For this review, take the finished solid that the model builds, in its own axes (mm). Face numbers are marked on the shaded views. A direction names the side the tool comes from. Round coordinates to 2 decimals unless told otherwise and drop trailing zeros. Loops run counter-clockwise (first coordinate to the right, second up) from the corner with the lowest first, then second, coordinate; pieces in that order, holes last. Notation, with made-up numbers: (-39, -3) -> (-26, -3) arc R26 cw to (-26, 14) -> close; hole circle Ø8 at (65, 25). An arc over 180 degrees is marked (long way). One line per question, with ' | ' between items. Start each with the question number.
1. For the marked faces 1, 2, 3 and 4, list the 3-axis set-ups (+Z, -Z, +X, -X, +Y, -Y) from which the entire face can be reached by the end or side of a thin tool; tool diameter is ignored.
2. Consider section B-B (z = 45). Write out the cut boundary in (x, y), and give its area (3 significant figures).
3. Consider section D-D (y = 25.5). Write out the cut boundary in (x, z), and give its area (3 significant figures).
4. Consider section A-A (y = 78). Write out the cut boundary in (x, z), and give its area (3 significant figures).
5. Wall thickness on line 1 along Z through (x, y) = (-76, 15.5); line 2 along X through (y, z) = (-24, 123); line 3 along Y through (x, z) = (-68, 65.5): over which ranges is each line inside the solid? List them lowest first.
6. For pin 1 Ø10 at (y, z) = (64.5, 103.5) entering from +X; pin 2 Ø4.5 at (x, y) = (-5.5, 86) entering from -Z; pin 3 Ø5 at (y, z) = (56.5, 121.5) entering from -X, all flat-tipped, find the tip position at first contact; note any pin that passes through.
7. Consider section C-C (z = 67.5). Write out the cut boundary in (x, y), and give its area (3 significant figures).
```python
from build123d import *

# Parameters (mm, degrees)
BOSS_EXTRUDE1_DEPTH = 150
BOSS_EXTRUDE2_REACH = 243.582
SKETCH2_W           = 54.603647952
SKETCH2_H           = 44.432380196
BOSS_EXTRUDE3_REACH = 243.582
SKETCH2_3_W         = 54.603647952
SKETCH2_3_H         = 44.432380196
MIRROR1_START       = 47.698176024
MIRROR1_DEPTH       = 54.603647952
CUT_EXTRUDE1_DEPTH  = 194.302477267
CUT_EXTRUDE2_DEPTH  = 54.603647952
BOSS_EXTRUDE4_START = -100
BOSS_EXTRUDE4_DEPTH = 10


# Read off the part's stored shape, not the designer's step: Mirror1
with BuildPart() as part:
    # Sketch1 → Boss-Extrude1 (new body)
    with BuildSketch(Plane.XY):
        Polygon((-42.309401077, 73.282032303), (-84.618802154, 0), (-63.464101615, -36.641016151), (-60, -34.641016151), (-80, 0), (-40, 69.282032303), (40, 69.282032303), (80, 0), (60, -34.641016151), (63.464101615, -36.641016151), (84.618802154, 0), (42.309401077, 73.282032303), align=None)
    extrude(amount=BOSS_EXTRUDE1_DEPTH)

    # Boss-Extrude2: up to this face of the body (flat: up to its plane)
    boss_extrude2_end = Plane(part.part.faces().sort_by_distance((74.041451884, -18.320508076, 75))[0])
    # Sketch2 → Boss-Extrude2 (add, up to the picked face)
    with BuildSketch(Plane(origin=(90, 0, 0), x_dir=(0, 0, -1), z_dir=(1, 0, 0)), mode=Mode.PRIVATE) as boss_extrude2_sk1:
        with Locations((-75, 0)):
            Rectangle(SKETCH2_W, SKETCH2_H)
    boss_extrude2_tool1 = split(extrude(boss_extrude2_sk1.sketch, amount=-BOSS_EXTRUDE2_REACH, mode=Mode.PRIVATE), bisect_by=boss_extrude2_end, keep=Keep.BOTH, mode=Mode.PRIVATE)
    add(boss_extrude2_tool1.solids().sort_by(Axis((90, 0, 75), (-1, 0, 0)))[0])

    # Boss-Extrude3: up to this face of the body (flat: up to its plane)
    boss_extrude3_end = Plane(part.part.faces().sort_by_distance((63.464101615, 36.641016151, 75))[0])
    # Sketch2<3> → Boss-Extrude3 (add, up to the picked face)
    with BuildSketch(Plane(origin=(90, 0, 0), x_dir=(0, 0, -1), z_dir=(1, 0, 0)), mode=Mode.PRIVATE) as boss_extrude3_sk1:
        with Locations((-75, 0)):
            Rectangle(SKETCH2_3_W, SKETCH2_3_H)
    boss_extrude3_tool1 = split(extrude(boss_extrude3_sk1.sketch, amount=-BOSS_EXTRUDE3_REACH, mode=Mode.PRIVATE), bisect_by=boss_extrude3_end, keep=Keep.BOTH, mode=Mode.PRIVATE)
    add(boss_extrude3_tool1.solids().sort_by(Axis((90, 0, 75), (-1, 0, 0)))[0])

    # Mirror1 outline → Mirror1 (add)
    with BuildSketch(Plane.XY.offset(MIRROR1_START)):
        Polygon((97.445325487, -22.216190098), (90, -9.320508076), (90, -22.216190098), align=None)
        Polygon((-67.173476666, -22.216190098), (67.173476666, -22.216190098), (80, 0), (67.173476666, 22.216190098), (-67.173476666, 22.216190098), (-80, 0), align=None)
        Polygon((-90, -22.216190098), (-71.79227882, -22.216190098), (-84.618802154, 0), (-71.79227882, 22.216190098), (-90, 22.216190098), align=None)
    extrude(amount=MIRROR1_DEPTH)

    # Sketch3 → Cut-Extrude1 (cut, through all)
    with BuildSketch(Plane.XY.offset(150)):
        Polygon((80, 0), (60, -34.641016151), (-60, -34.641016151), (-80, 0), (-40, 69.282032303), (40, 69.282032303), align=None)
    extrude(amount=-CUT_EXTRUDE1_DEPTH, mode=Mode.SUBTRACT)

    # Sketch4 → Cut-Extrude2 (cut)
    with BuildSketch(Plane.XY.offset(102.301823976)):
        Polygon((90, -9.320508076), (90, -22.216190098), (97.445325487, -22.216190098), align=None)
    extrude(amount=-CUT_EXTRUDE2_DEPTH, mode=Mode.SUBTRACT)

    # Sketch5 → Boss-Extrude4 (add)
    with BuildSketch(Plane.XY.offset(150).offset(BOSS_EXTRUDE4_START)):
        with BuildLine():
            Line((-9.78911305, 73.282032303), (-9.78911305, 83.156762189))
            ThreePointArc((-9.78911305, 83.156762189), (-1.963791345, 90.982083893), (5.861530359, 83.156762189))
            Line((5.861530359, 83.156762189), (5.861530359, 73.282032303))
            Line((5.861530359, 73.282032303), (2.861530359, 73.282032303))
            Line((2.861530359, 73.282032303), (2.861530359, 83.156762189))
            ThreePointArc((2.861530359, 83.156762189), (-1.963791345, 87.982083893), (-6.78911305, 83.156762189))
            Line((-6.78911305, 83.156762189), (-6.78911305, 73.282032303))
            Line((-6.78911305, 73.282032303), (-9.78911305, 73.282032303))
        make_face()
    extrude(amount=-BOSS_EXTRUDE4_DEPTH)


solid = part.part
```
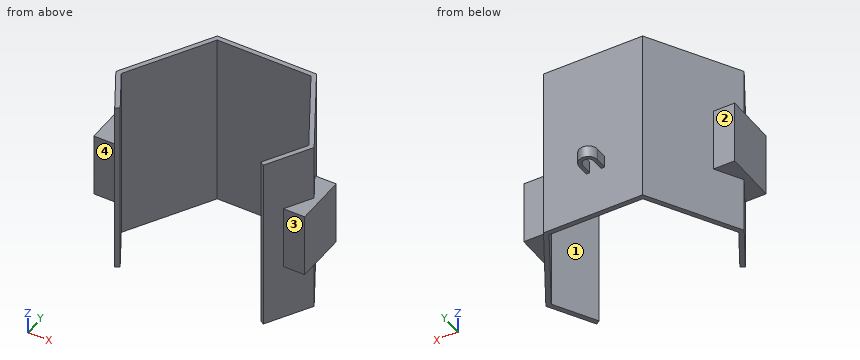
Answer block:
1) face 1: +Z, -Z | face 2: +Z, -Z, -X, +Y | face 3: +Z, -Z, +X, -Y | face 4: +Z, -Z, -X, -Y
2) outline: (-84.62, 0) -> (-63.46, -36.64) -> (-60, -34.64) -> (-80, 0) -> (-40, 69.28) -> (40, 69.28) -> (80, 0) -> (60, -34.64) -> (63.46, -36.64) -> (84.62, 0) -> (42.31, 73.28) -> (5.86, 73.28) -> (5.86, 83.16) arc R7.83 ccw to (-9.79, 83.16) -> (-9.79, 73.28) -> (-42.31, 73.28) -> close; hole (-6.79, 73.28) -> (2.86, 73.28) -> (2.86, 83.16) arc R4.83 ccw to (-6.79, 83.16) -> close | area: 1,440 mm2
3) outline: (-69.9, 0) -> (-65.28, 0) -> (-65.28, 150) -> (-69.9, 150) -> close; (65.28, 0) -> (69.9, 0) -> (69.9, 150) -> (65.28, 150) -> close | area: 1,390 mm2
4) outline: (-9.79, 40) -> (-6.79, 40) -> (-6.79, 50) -> (-9.79, 50) -> close; (2.86, 40) -> (5.86, 40) -> (5.86, 50) -> (2.86, 50) -> close | area: 60.0 mm2
5) line 1: z = 47.7 to 102.3 | line 2: x = -70.76 to -66.14, 66.14 to 70.76 | line 3: y = -28.78 to -20.78, 20.78 to 28.78
6) pin 1: stops at x = 50.27 | pin 2: stops at z = 40 | pin 3: stops at x = -53.44
7) outline: (-90, -22.22) -> (-71.79, -22.22) -> (-63.46, -36.64) -> (-60, -34.64) -> (-80, 0) -> (-40, 69.28) -> (40, 69.28) -> (80, 0) -> (60, -34.64) -> (63.46, -36.64) -> (71.79, -22.22) -> (90, -22.22) -> (90, 22.22) -> (71.79, 22.22) -> (42.31, 73.28) -> (-42.31, 73.28) -> (-71.79, 22.22) -> (-90, 22.22) -> close | area: 2,370 mm2
